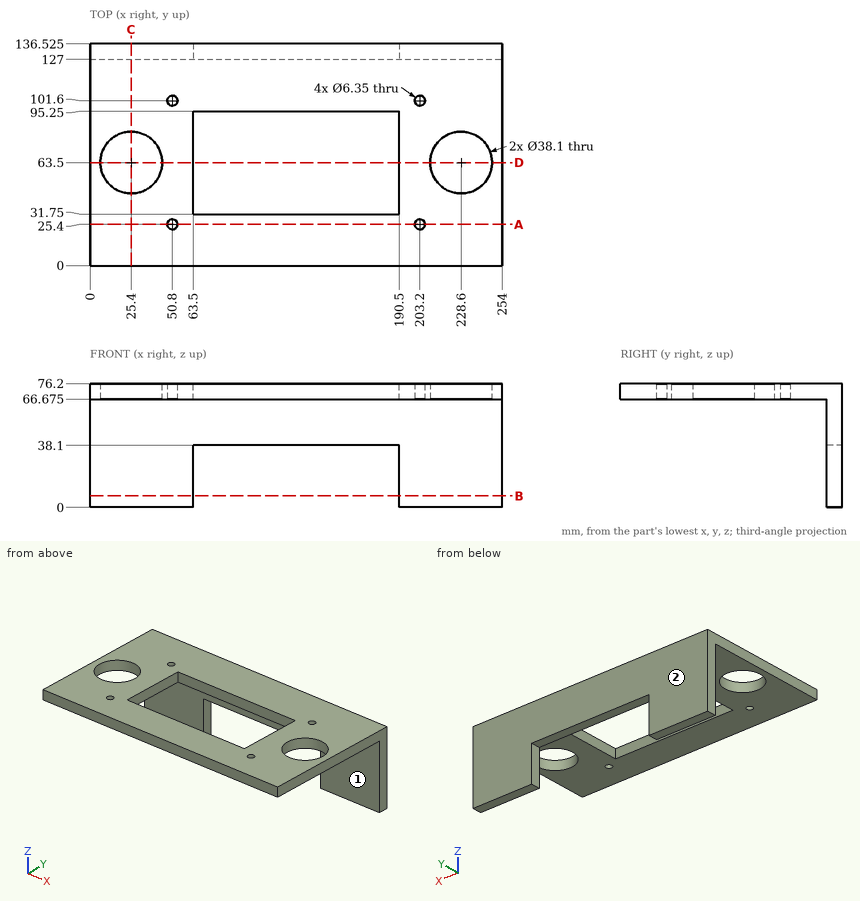
The figure shows three views and two pictorial views of one solid part (mm, origin at its lowest corner). Answer the questions. A direction names the side the tool comes from. Round coordinates to 2 decimals unless told otherwise and drop trailing zeros. Write each loop counter-clockwise with the first axis right and the second up, starting at its lowest first coordinate (ties: lowest second). Pieces come first, ordered by that corner, then holes. Notation, with made-up numbers: (58.5, 38.5) -> (91.5, 38.5) arc R17 ccw to (91.5, 70.5) -> close; hole circle Ø5 at (-26.75, -1.5). An arc over 180 degrees is marked (long way). Answer as a JSON object with one key per item and string values. Group by question number.
Q1. Section D-D (y = 63.5) is taken. Write down the section's boundary in (x, z) (3 decimals), plus the area to 3 significant figures.
Q2. Each of these flat-tipped pins is pushed along its axis until it touches: pin 1 Ø6 at (y, z) = (121.5, 26.5) entering from +X; pin 2 Ø4 at (x, y) = (27, 111) entering from -Z (3 decimals); pin 3 Ø3 at (y, z) = (131.5, 13.5) entering from -X; pin 4 Ø10 at (x, z) = (63, 55.5) entering from -Y. Where does it stop, or does it pass through?
Q3. Straight lines are drawn through the part: line 1 along X through (y, z) = (101.6, 69) (3 decimals); line 2 along X through (y, z) = (25, 69); line 3 along X through (y, z) = (63.5, 73.75). For each, find the intervals that lie inside material, in ascending order.
Q4. Section A-A (y = 25.4) is taken. Write down the section's boundary in (x, z) (3 decimals).
Q5. Which of the six approach directions +Z, -Z, +X, -X, +Y, -Y give full straight-line access (tool end or side, diameter ignored) to the marked faces 1 and 2?
Q6. Section C-C (x = 25.4) is taken. Write down the section's boundary in (y, z) (3 decimals), plus the area to 3 significant figures.
Q7. Section B-B (z = 7) is taken. Write down the section's boundary in (x, y) (3 decimals), plus the area to 3 significant figures.
Check values:
{
 "1": {"outline": "(0, 66.675) -> (6.35, 66.675) -> (6.35, 76.2) -> (0, 76.2) -> close; (44.45, 66.675) -> (63.5, 66.675) -> (63.5, 76.2) -> (44.45, 76.2) -> close; (190.5, 66.675) -> (209.55, 66.675) -> (209.55, 76.2) -> (190.5, 76.2) -> close; (247.65, 66.675) -> (254, 66.675) -> (254, 76.2) -> (247.65, 76.2) -> close", "area": "484 mm^2"},
 "2": {"pin 1": "through", "pin 2": "z = 66.675", "pin 3": "x = 0", "pin 4": "y = 127"},
 "3": {"line 1": "0 to 47.625, 53.975 to 200.025, 206.375 to 254", "line 2": "0 to 47.65, 53.95 to 200.05, 206.35 to 254", "line 3": "0 to 6.35, 44.45 to 63.5, 190.5 to 209.55, 247.65 to 254"},
 "4": {"outline": "(0, 66.675) -> (47.625, 66.675) -> (47.625, 76.2) -> (0, 76.2) -> close; (53.975, 66.675) -> (200.025, 66.675) -> (200.025, 76.2) -> (53.975, 76.2) -> close; (206.375, 66.675) -> (254, 66.675) -> (254, 76.2) -> (206.375, 76.2) -> close"},
 "5": {"face 1": "-Z, +X, -X, -Y", "face 2": "+Z, -Z, +X, -X, +Y"},
 "6": {"outline": "(0, 66.675) -> (44.45, 66.675) -> (44.45, 76.2) -> (0, 76.2) -> close; (82.55, 66.675) -> (127, 66.675) -> (127, 0) -> (136.525, 0) -> (136.525, 76.2) -> (82.55, 76.2) -> close", "area": "1,570 mm^2"},
 "7": {"outline": "(0, 127) -> (63.5, 127) -> (63.5, 136.525) -> (0, 136.525) -> close; (190.5, 127) -> (254, 127) -> (254, 136.525) -> (190.5, 136.525) -> close", "area": "1,210 mm^2"}
}
